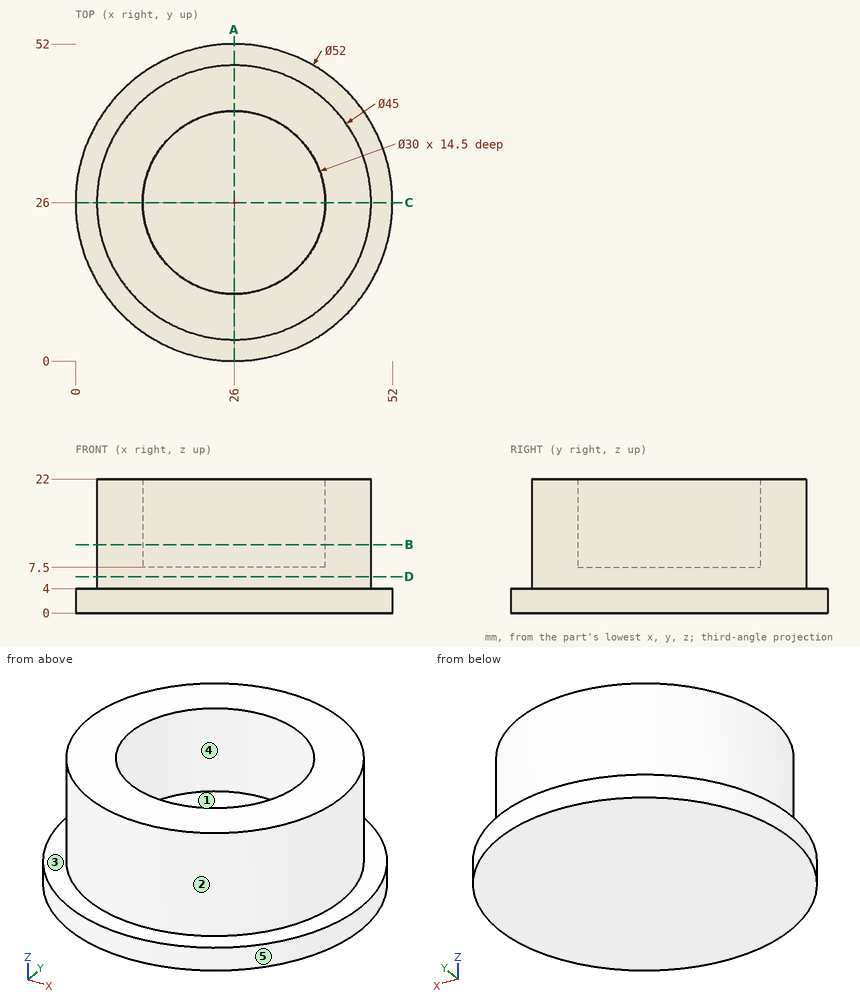
Source: three-view drawing plus pictorial views. Frame: mm from the lowest corner of the part. A direction names the side the tool comes from. Round coordinates to 2 decimals unless told otherwise and drop trailing zeros. Loops run counter-clockwise (first coordinate to the right, second up) from the corner with the lowest first, then second, coordinate; pieces in that order, holes last.
Item 1: Line query: L1, parallel to Y at x = 26, z = 17.25; L2, parallel to Z at x = 48, y = 32.5; L3, parallel to Y at x = 38, z = 12.75. Output: solid intervals per line, ascending.
Checked values:
L1: y = 3.5 to 11, 41 to 48.5
L2: z = 0 to 4
L3: y = 6.97 to 17, 35 to 45.03
Item 2: Section A-A, the plane x = 26. Output: boundary loops of the cut face in (y, z).
Checked values:
outline: (0, 0) - (52, 0) - (52, 4) - (48.5, 4) - (48.5, 22) - (41, 22) - (41, 7.5) - (11, 7.5) - (11, 22) - (3.5, 22) - (3.5, 4) - (0, 4) - close
Item 3: Contact query for flat-ended pins moving along their axis: P1, Ø3, axis at x = 6, y = 43.5, coming from the -Z side; P2, Ø12, axis at x = 37, z = 17, coming from the +Y side; P3, Ø10, axis at y = 5.5, z = 17.5, coming from the -X side; P4, Ø4, axis at x = 20.5, z = 13.5, coming from the -Y side. Output: stop coordinate, or through.
Checked values:
P1: stops at z = 0
P2: stops at y = 47.94
P3: stops at x = 9.69
P4: stops at y = 3.77
Item 4: Section B-B, the plane z = 11.25. Output: boundary loops of the cut face in (x, y).
Checked values:
outline: circle Ø45 at (26, 26); hole circle Ø30 at (26, 26)
Item 5: Mould query, pull axis X, two halves, no side actions, for the marked faces 1, 2 and 3. Classes: released by +X, released by -X, zero draft, split by the parting line, or undercut.
Checked values:
face 1: undercut
face 2: split by the parting line
face 3: zero draft
Item 6: Section D-D, the plane z = 6. Output: boundary loops of the cut face in (x, y).
Checked values:
outline: circle Ø45 at (26, 26)
Item 7: Reachability of the marked faces 4 and 5 from +Z, -Z, +X, -X, +Y, -Y: full face, straight path, thin tool, end or side. Return the list, or none.
Checked values:
face 4: +Z
face 5: +Z, -Z
